```python
from build123d import *

# Parameters (mm, degrees)
IZIM1_R                     = 15
Y_KSEKLIK_EKSTR_ZYON1_DEPTH = 5
Y_KSEKLIK_EKSTR_ZYON2_DEPTH = 5
IZIM3_R                     = 4
KES_EKSTR_ZYON1_DEPTH       = 11


with BuildPart() as part:
    # Çizim1 → Yükseklik-Ekstrüzyon1 (new body, symmetric)
    with BuildSketch(Plane.XY):
        Circle(IZIM1_R)
    extrude(amount=Y_KSEKLIK_EKSTR_ZYON1_DEPTH, both=True)

    # Çizim2 → Yükseklik-Ekstrüzyon2 (add, symmetric)
    with BuildSketch(Plane.XY):
        Polygon((-2, 13.2), (2, 13.2), (0.5, 17.321216129), (-0.5, 17.321216129), align=None)
        Polygon((4.877021889, 16.627963967), (2.176911293, 13.171980004), (5.981137358, 11.935912026), (5.828078405, 16.318946973), align=None)
        Polygon((9.776646895, 14.307050838), (6.140731342, 11.85459483), (9.376799319, 9.503453821), (10.58566389, 13.719265586), align=None)
        Polygon((13.719265586, 10.58566389), (9.503453821, 9.376799319), (11.85459483, 6.140731342), (14.307050838, 9.776646895), align=None)
        Polygon((16.318946973, 5.828078405), (11.935912026, 5.981137358), (13.171980004, 2.176911293), (16.627963967, 4.877021889), align=None)
        Polygon((17.321216129, 0.5), (13.2, 2), (13.2, -2), (17.321216129, -0.5), align=None)
        Polygon((16.627963967, -4.877021889), (13.171980004, -2.176911293), (11.935912026, -5.981137358), (16.318946973, -5.828078405), align=None)
        Polygon((14.307050838, -9.776646895), (11.85459483, -6.140731342), (9.503453821, -9.376799319), (13.719265586, -10.58566389), align=None)
        Polygon((10.58566389, -13.719265586), (9.376799319, -9.503453821), (6.140731342, -11.85459483), (9.776646895, -14.307050838), align=None)
        Polygon((5.828078405, -16.318946973), (5.981137358, -11.935912026), (2.176911293, -13.171980004), (4.877021889, -16.627963967), align=None)
        Polygon((0.5, -17.321216129), (2, -13.2), (-2, -13.2), (-0.5, -17.321216129), align=None)
        Polygon((-4.877021889, -16.627963967), (-2.176911293, -13.171980004), (-5.981137358, -11.935912026), (-5.828078405, -16.318946973), align=None)
        Polygon((-9.776646895, -14.307050838), (-6.140731342, -11.85459483), (-9.376799319, -9.503453821), (-10.58566389, -13.719265586), align=None)
        Polygon((-13.719265586, -10.58566389), (-9.503453821, -9.376799319), (-11.85459483, -6.140731342), (-14.307050838, -9.776646895), align=None)
        Polygon((-16.318946973, -5.828078405), (-11.935912026, -5.981137358), (-13.171980004, -2.176911293), (-16.627963967, -4.877021889), align=None)
        Polygon((-17.321216129, -0.5), (-13.2, -2), (-13.2, 2), (-17.321216129, 0.5), align=None)
        Polygon((-16.627963967, 4.877021889), (-13.171980004, 2.176911293), (-11.935912026, 5.981137358), (-16.318946973, 5.828078405), align=None)
        Polygon((-14.307050838, 9.776646895), (-11.85459483, 6.140731342), (-9.503453821, 9.376799319), (-13.719265586, 10.58566389), align=None)
        Polygon((-10.58566389, 13.719265586), (-9.376799319, 9.503453821), (-6.140731342, 11.85459483), (-9.776646895, 14.307050838), align=None)
        Polygon((-5.828078405, 16.318946973), (-5.981137358, 11.935912026), (-2.176911293, 13.171980004), (-4.877021889, 16.627963967), align=None)
    extrude(amount=Y_KSEKLIK_EKSTR_ZYON2_DEPTH, both=True)

    # Çizim3 → Kes-Ekstrüzyon1 (cut, through all)
    with BuildSketch(Plane(origin=(0, 0, -5), x_dir=(-1, 0, 0), z_dir=(0, 0, -1))):
        Circle(IZIM3_R)
    extrude(amount=-KES_EKSTR_ZYON1_DEPTH, mode=Mode.SUBTRACT)


solid = part.part
```
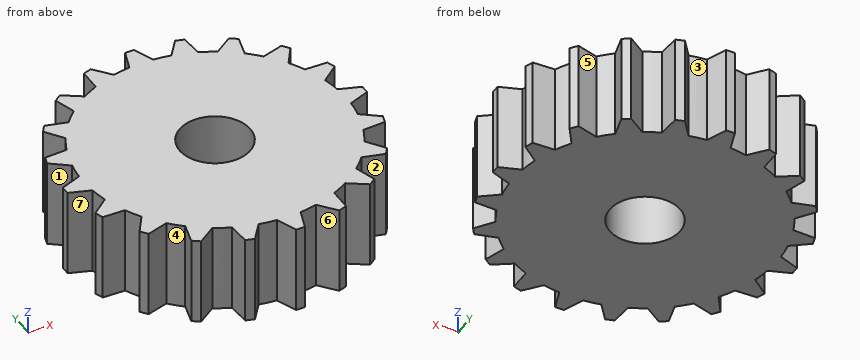
Model file for the job. Use its own axes, mm. Face numbers are marked on the shaded views. A direction names the side the tool comes from. Coordinates: 2 decimals unless noted, no trailing zeros. Order: outer loops, then holes, each group sorted by start corner. A loop starts at its lowest first (then second) coordinate and runs counter-clockwise, first axis right, second up. Notation, with made-up numbers: (70.25, 28.5) - (108.25, 28.5) arc R23 cw to (108.25, 55.5) - close; hole circle Ø1 at (6, -19). An arc over 180 degrees is marked (long way). Return JSON: item names as keys, results as strings. Group by question number.
1) Saw through at A-A, the plane y = 0. Write the cut outline in (x, z).
2) Probe line 1 (Y direction, x = 0, z = 2); line 2 (X direction, y = -14, z = 2); line 3 (X direction, y = -13, z = 2). List the from-to ranges inside material, lowest first. Write a range as from..to.
3) Flat gauge pins, fed straight in: P1, Ø1.5, axis at y = -5.5, z = 1.5, coming from the -X side; P2, Ø5, axis at x = -10, z = -2, coming from the +Y side; P3, Ø1, axis at y = 3, z = -0.5, coming from the -X side; P4, Ø7, axis at x = 0, y = 0, coming from the -Z side. Where does each tip first touch, or does it go through?
4) Mould opens along Y. For the marked faces 1, 2 and 3 say: released by +Y, released by -Y, zero draft, split by the parting line, or undercut.
5) Tool access for the marked faces 4, 5, 6 and 7: list every direction of +Z, -Z, +X, -X, +Y, -Y with a clear straight run to the whole face (end or side of a thin tool).
Values found:
{
 "1": {"outline": "(-17.32, -5) - (-4, -5) - (-4, 5) - (-17.32, 5) - close; (4, -5) - (17.32, -5) - (17.32, 5) - (4, 5) - close"},
 "2": {"line 1": "y = -17.32..-4, 4..17.32", "line 2": "x = -10.2..-9.32, -5.91..5.91, 9.32..10.2", "line 3": "x = -10.38..-7.84, -7.48..7.48, 7.84..10.38"},
 "3": {"P1": "stops at x = -16.63", "P2": "stops at y = 14.31", "P3": "stops at x = -14.87", "P4": "passes through"},
 "4": {"face 1": "undercut", "face 2": "released by -Y", "face 3": "released by +Y"},
 "5": {"face 4": "+Z, -Z", "face 5": "+Z, -Z, +Y", "face 6": "+Z, -Z, -Y", "face 7": "+Z, -Z, -X"}
}
